The listing builds one solid part. Answer for the finished solid, in the listing's coordinates (mm). A direction names the side the tool comes from. Round coordinates to 2 decimals unless told otherwise and drop trailing zeros. Write each loop counter-clockwise with the first axis right and the second up, starting at its lowest first coordinate (ties: lowest second). Pieces come first, ordered by that corner, then holes. Notation, with made-up numbers: (-35, 6) - (-4, 6) arc R23 cw to (-4, 21) - close; hole circle Ø7 at (81, -6). An arc over 180 degrees is marked (long way). Return JSON: item names as keys, results as strings. Group by question number.
(1) Section A-A, the plane y = 62.35 is taken. Write down the section's boundary in (x, z).
(2) Section C-C, the plane y = 0 is taken. Write down the section's boundary in (x, z).
(3) Section B-B, the plane z = 16 is taken. Write down the section's boundary in (x, y), then the cut area to 3 significant figures.
(4) Which of the six approach directions +Z, -Z, +X, -X, +Y, -Y give full straight-line access (tool end or side, diameter ignored) to faces 1 (the flat face through (16.6, 31, 1)), 2 (the flat face through (-16.6, -31, 1)), 3 (the flat face through (0, -12.5, 11)), 4 (the cylindrical face through (12.5, 0.2, 9.9))?
(5) Find the intervals of material crossed by line 1 along Y through (x, z) = (-20.4, 1.7); line 2 along Y through (x, z) = (3, 5), in increasing order. Write a range as [from, to].
(6) Each of these flat-tipped pins is pushed along its axis until it touches: pin 1 (1.5 mm diameter, centred on x = -12.5, y = -26, fed in from +Z); pin 2 (10 mm diameter, centred on x = -4.5, z = 9, fed in from +Y); pin 3 (1.4 mm diameter, centred on y = 29, z = 2, fed in from +X); pin 4 (5.5 mm diameter, centred on x = 20.4, y = 62.35, fed in from -Z). Where does it stop, or does it pass through?
(7) Determine the mould class of faces 5 (the cylindrical face through (-19.27, -64.12, 1.36)), 6 (the flat face through (0, 12.5, 11)), 7 (the flat face through (0, -67.25, 1)) for opening direction Y: +Y half, -Y half, draft (parallel to the pull), parting line (faces both ways), or undercut.
(8) Section D-D, the plane x = 0 is taken. Write down the section's boundary in (y, z), then the cut area to 3 significant figures.
Autodesk Inventor part; units mm, degrees
ref_plane "Work Plane1" through (0, 0, 52.75) normal (0, 0, 1) x (1, 0, 0)
ref_plane "YZ Plane" through (0, 0, 0) normal (1, 0, 0) x (0, 1, 0)
ref_plane "XZ Plane" through (0, 0, 0) normal (0, 1, 0) x (-1, 0, 0)
sketch "Sketch1" plane through (0, 0, 0) normal (0, 0, 1) x (1, 0, 0)
  line L0 (-8.124, 9.5) -> (8.124, 9.5)
  line L1 (-8.124, -9.5) -> (8.124, -9.5)
  line L2 (-14.5312, 0) -> (9.3904, 0) construction
  arc A0 (-8.124, 9.5) -> (-8.124, -9.5) centre (0, 0) ccw
  arc A1 (8.124, -9.5) -> (8.124, 9.5) centre (0, 0) ccw
  line L3 (-29.5712, -67.25) -> (29.5712, -67.25)
  line L4 (29.5712, 67.25) -> (-29.5712, 67.25)
  arc A2 (-20.4, -57.45) -> (-20.4, -67.25) centre (-20.4, -62.35) ccw
  line L5 (-20.4, -67.25) -> (-29.5712, -67.25)
  line L6 (-20.4, -57.45) -> (-16.6, -57.45)
  circle A3 centre (-20.4, -62.35) radius 2.1
  line L7 (0, -40.5988) -> (0, 24.1265) construction
  arc A4 (-20.4, 67.25) -> (-20.4, 57.45) centre (-20.4, 62.35) ccw
  line L8 (-20.4, 67.25) -> (-29.5712, 67.25)
  line L9 (-20.4, 57.45) -> (-16.6, 57.45)
  circle A5 centre (-20.4, 62.35) radius 2.1
  arc A6 (20.4, -67.25) -> (20.4, -57.45) centre (20.4, -62.35) ccw
  line L10 (20.4, -67.25) -> (29.5712, -67.25)
  line L11 (20.4, -57.45) -> (16.6, -57.45)
  circle A7 centre (20.4, -62.35) radius 2.1
  line L12 (20.4, 57.45) -> (16.6, 57.45)
  circle A8 centre (20.4, 62.35) radius 2.1
  line L13 (20.4, 67.25) -> (29.5712, 67.25)
  arc A9 (20.4, 57.45) -> (20.4, 67.25) centre (20.4, 62.35) ccw
  arc A10 (-20.4, 4.9) -> (-20.4, -4.9) centre (-20.4, 0) ccw
  line L14 (-20.4, -4.9) -> (-16.6, -4.9)
  line L15 (-20.4, 4.9) -> (-16.6, 4.9)
  circle A11 centre (-20.4, 0) radius 2.1
  line L16 (-16.6, 57.45) -> (-16.6, 4.9)
  line L17 (-16.6, -4.9) -> (-16.6, -57.45)
  line L18 (20.4, 4.9) -> (16.6, 4.9)
  arc A12 (20.4, -4.9) -> (20.4, 4.9) centre (20.4, 0) ccw
  circle A13 centre (20.4, 0) radius 2.1
  line L19 (20.4, -4.9) -> (16.6, -4.9)
  line L20 (16.6, -57.45) -> (16.6, -4.9)
  line L21 (16.6, 4.9) -> (16.6, 57.45)
  line L22 (9.1652, -12.5) -> (-9.1652, -12.5)
  arc A14 (-9.1652, 12.5) -> (-9.1652, -12.5) centre (0, 0) ccw
  line L23 (-9.1652, 12.5) -> (9.1652, 12.5)
  arc A15 (9.1652, -12.5) -> (9.1652, 12.5) centre (0, 0) ccw
  point P0 (-42.7024, 0)
  dimension "d1" = 19
  dimension "d2" = 4.2
  dimension "d3" = 4.9
  dimension "d4" = 134.5
  dimension "d5" = 4.2
  dimension "d6" = 4.9
  dimension "d9" = 3
  dimension "d34" = 33.2
  dimension "d35" = 3.8
  dimension "d36" = 3.8
  dimension "d37" = 12.5
  dimension "d38" = 12.5
extrude "Extrusion1" add sketch "Sketch1" along normal blind 2.75 contours A2 L6 L17 L14 A10 L15 L16 L9 A4 L4 A9 L12 L21 L18 A12 L19 L20 L11 A6 L3 | L22 A14 L23 A15
extrude "Extrusion2" add sketch "Sketch1" along normal blind 20 contours L22 A14 L23 A15
ref_plane "Work Plane1" through (0, 0, 52.75) normal (0, 0, 1) x (1, 0, 0)
properties part number "Gripper_MotorHolder"
Working result:
{
 "1": {"outline": "(-25.3, 0) - (-22.5, 0) - (-22.5, 2.75) - (-25.3, 2.75) - close; (-18.3, 0) - (18.3, 0) - (18.3, 2.75) - (-18.3, 2.75) - close; (22.5, 0) - (25.3, 0) - (25.3, 2.75) - (22.5, 2.75) - close"},
 "2": {"outline": "(-25.3, 0) - (-22.5, 0) - (-22.5, 2.75) - (-25.3, 2.75) - close; (-18.3, 0) - (-12.5, 0) - (-12.5, 20) - (-15.5, 20) - (-15.5, 2.75) - (-18.3, 2.75) - close; (12.5, 0) - (18.3, 0) - (18.3, 2.75) - (15.5, 2.75) - (15.5, 20) - (12.5, 20) - close; (22.5, 0) - (25.3, 0) - (25.3, 2.75) - (22.5, 2.75) - close"},
 "3": {"outline": "(-9.17, -12.5) - (9.17, -12.5) arc R15.5 ccw to (9.17, 12.5) - (-9.17, 12.5) arc R15.5 ccw to start; hole (-8.12, -9.5) - (8.12, -9.5) arc R12.5 ccw to (8.12, 9.5) - (-8.12, 9.5) arc R12.5 ccw to start", "area": "256 mm^2"},
 "4": {"face 1": "+Z, -Z, +X", "face 2": "+Z, -Z, -X", "face 3": "+Z, +X, -X, -Y", "face 4": "+Z, -Z"},
 "5": {"line 1": "y = [-67.25, -64.45], [-60.25, -57.45], [-4.9, -2.1], [2.1, 4.9], [57.45, 60.25], [64.45, 67.25]", "line 2": "y = [-12.5, -9.5], [9.5, 12.5]"},
 "6": {"pin 1": "stops at z = 2.75", "pin 2": "stops at y = 12.5", "pin 3": "stops at x = 16.6", "pin 4": "stops at z = 0"},
 "7": {"face 5": "undercut", "face 6": "+Y half", "face 7": "-Y half"},
 "8": {"outline": "(-67.25, 0) - (-9.5, 0) - (-9.5, 20) - (-12.5, 20) - (-12.5, 2.75) - (-67.25, 2.75) - close; (9.5, 0) - (67.25, 0) - (67.25, 2.75) - (12.5, 2.75) - (12.5, 20) - (9.5, 20) - close", "area": "421 mm^2"}
}
